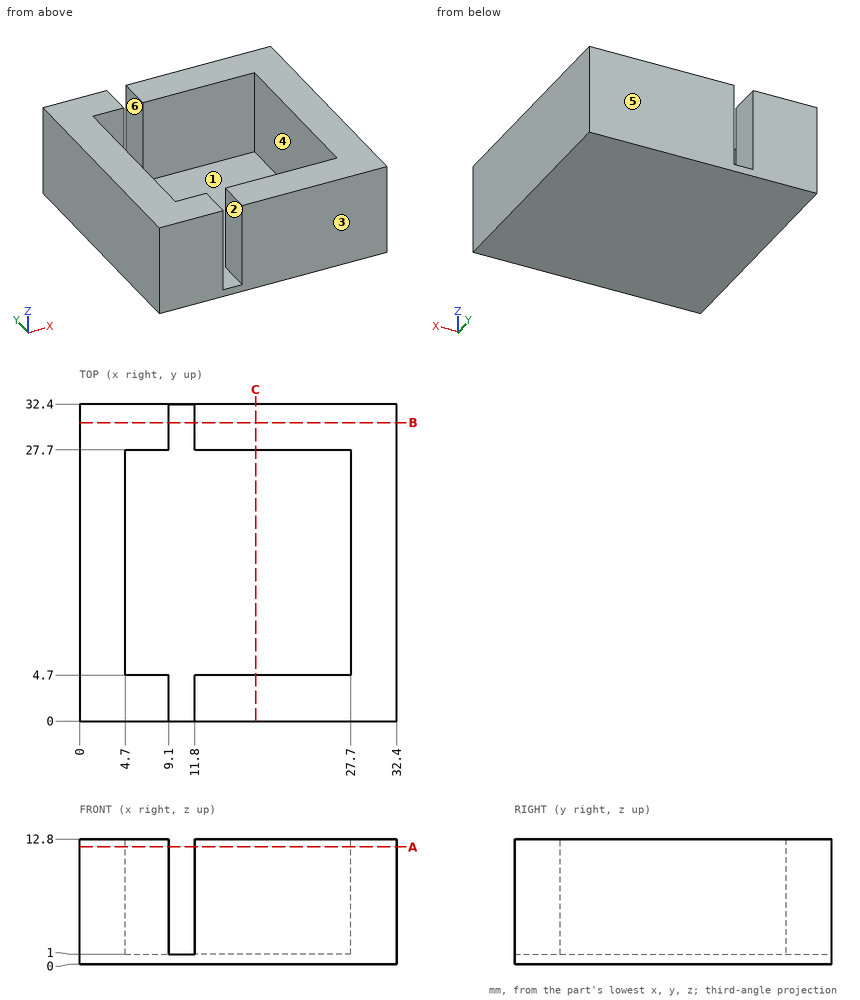
Here's the drawing with two shaded views (mm, measured from the low corner). I have some questions. A direction names the side the tool comes from. Give positions to 0.01 mm unless a question says otherwise; leave off trailing zeros. Loops run counter-clockwise (first coordinate to the right, second up) from the corner with the lowest first, then second, coordinate; pieces in that order, holes last. Notation, with made-up numbers: M -22.5,36 L -6.5,36 A26 cw -6.5,72 Z; hole C -31.5,76 d6. An arc over 180 degrees is marked long. Use one line per item in the form item = value. Start each with the question number.
(1) Thinking about a two-plate mould opening in Y: for the marked faces 1, 2 and 3, which applies, released by +Y, released by -Y, zero draft, split by the parting line, or undercut?
(2) I want a section at B-B, the plane y = 30.5. Write out the boundary of the cut face in (x, z), and give its area (3 significant figures).
(3) On a 3-axis mill with a long thin cutter (end or side, diameter ignored), from which of +Z, -Z, +X, -X, +Y, -Y can I reach the whole of each face in a straight line? I mean the marked faces 4, 5 and 6. Say none if no direction works.
(4) I want a section at A-A, the plane z = 12. Write out the boundary of the cut face in (x, y).
(5) I want a section at C-C, the plane x = 18. Write out the boundary of the cut face in (y, z), and give its area (3 significant figures).
(6) I'm going to push a flat-ended pin straight in: P1, Ø10, axis at x = 18, y = 18.5, coming from the +Z side. Where does the tip first touch, or does it pass through?
(7) Please list where these lines run through material, in increasing order: line 1 (X direction, y = 7.5, z = 8); line 2 (X direction, y = 28.5, z = 4.75).
Worked out:
q1.face_1 = undercut
q1.face_2 = zero draft
q1.face_3 = released by -Y
q2.outline = M 0,0 L 32.4,0 L 32.4,12.8 L 11.8,12.8 L 11.8,1 L 9.1,1 L 9.1,12.8 L 0,12.8 Z
q2.area = 383 mm²
q3.face_4 = +Z
q3.face_5 = +Z, -Z, +X, -X, +Y
q3.face_6 = +Z, +Y, -Y
q4.outline = M 0,0 L 9.1,0 L 9.1,4.7 L 4.7,4.7 L 4.7,27.7 L 9.1,27.7 L 9.1,32.4 L 0,32.4 Z; M 11.8,0 L 32.4,0 L 32.4,32.4 L 11.8,32.4 L 11.8,27.7 L 27.7,27.7 L 27.7,4.7 L 11.8,4.7 Z
q5.outline = M 0,0 L 32.4,0 L 32.4,12.8 L 27.7,12.8 L 27.7,1 L 4.7,1 L 4.7,12.8 L 0,12.8 Z
q5.area = 143 mm²
q6.P1 = 1
q7.line_1 = 0 to 4.7, 27.7 to 32.4
q7.line_2 = 0 to 9.1, 11.8 to 32.4
